Source: CAD feature listing. Evaluate the final solid. Frame: model axes, mm. Face numbers are marked on the shaded views. A direction names the side the tool comes from. Give positions to 0.01 mm unless a question says otherwise; leave off trailing zeros. Order: outer loops, then holes, each group sorted by start corner. A loop starts at its lowest first (then second) coordinate and runs counter-clockwise, first axis right, second up. Notation, with made-up numbers: M -11,50.25 L 17,50.25 A19 ccw 17,61.25 Z; hole C -31,48 d8. An arc over 180 degrees is marked long. Answer as a JSON object with one key per item and string values. Group by question number.
1. Section query B-B (x = 0). Output: boundary loops of the cut face in (y, z).
2. Pin query (flat end, axial travel): P1, Ø3, axis at x = -27, z = -22, coming from the +Y side; P2, Ø6, axis at x = 7, y = 9.5, coming from the -Z side; P3, Ø2, axis at x = 7, y = 5.5, coming from the +Z side. Return the tip coordinate at first contact, or that it passes through.
3. Section query A-A (z = 0). Output: boundary loops of the cut face in (x, y).
4. Pull-direction query (Z, two-part tool) for the marked faces 3, 4 and 5; classes: +Z half, -Z half, draft (parallel to the pull), parting line (faces both ways), or undercut.
5. Set-up query: the marked faces 1 and 2. Return all of +Z, -Z, +X, -X, +Y, -Y with unobstructed straight access to the full face (end or side cutting, diameter ignored); none if empty.
6. Section query C-C (y = 9.5). Output: boundary loops of the cut face in (x, z), plus the area to 3 significant figures.
7. Material intervals for L1, parallel to X at y = 4.25, z = -0.5; L2, parallel to Y at x = 19.5, z = 22; L3, parallel to Z at x = 7, y = 7.75, sorted ascending. Write a range as [from, to].
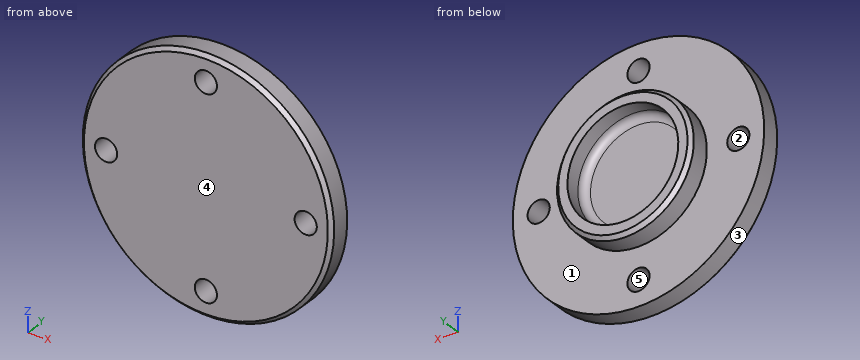
from build123d import *

# Parameters (mm, degrees)
SKETCH_1_R               = 34
EXTRUDE_1_DEPTH          = 6
SKETCH_2_R               = 18.5
SKETCH_2_R_2             = 15
EXTRUDE_2_DEPTH          = 6
SKETCH_5_R               = 3
CUT_EXTRUDE_1_DEPTH      = 6
PATTERN_CIRCULAR_1_COUNT = 4
FILLET_1_R               = 2
CHAMFER_1_SIZE           = 1


with BuildPart() as part:
    # 草图1 → 凸台-拉伸1 (new body)
    with BuildSketch(Plane(origin=(0, 0, 0), x_dir=(1, 0, 0), z_dir=(0, 1, 0))):
        with Locations(Location((0, 0, 0), (0, 0, 270))):
            Circle(SKETCH_1_R)
    extrude(amount=EXTRUDE_1_DEPTH)

    # 草图2 → 凸台-拉伸2 (add)
    with BuildSketch(Plane(origin=(0, 6, 0), x_dir=(1, 0, 0), z_dir=(0, 1, 0))):
        with Locations(Location((0, 0, 0), (0, 0, 270))):
            Circle(SKETCH_2_R)
        with Locations(Location((0, 0, 0), (0, 0, 270))):
            Circle(SKETCH_2_R_2, mode=Mode.SUBTRACT)
    extrude(amount=EXTRUDE_2_DEPTH)

    # 草图5 → 切除-拉伸1 (cut)
    with BuildSketch(Plane(origin=(0, 6, 0), x_dir=(1, 0, 0), z_dir=(0, 1, 0))):
        with Locations(Location((0, 27, 0), (0, 0, 270))):
            Circle(SKETCH_5_R)
    cut_extrude_1 = extrude(amount=-CUT_EXTRUDE_1_DEPTH, mode=Mode.SUBTRACT)

    # 阵列(圆周)1: 切除-拉伸1 ×4 about axis
    pattern_circular_1_axis = Axis((0, 0, 0), (0, 1, 0))
    for i in range(1, PATTERN_CIRCULAR_1_COUNT):
        add(cut_extrude_1.rotate(pattern_circular_1_axis, i * 360 / PATTERN_CIRCULAR_1_COUNT), mode=Mode.SUBTRACT)

    # 圆角1
    fillet_1_edges = [part.edges().sort_by_distance(p)[0] for p in [
        (0, 6, -15),
    ]]
    fillet(fillet_1_edges, radius=FILLET_1_R)

    # 倒角1
    chamfer_1_edges = [part.edges().sort_by_distance(p)[0] for p in [
        (0, 12, -18.5),
        (0, 0, -34),
    ]]
    chamfer(chamfer_1_edges, length=CHAMFER_1_SIZE)


solid = part.part
Answer sheet:
{
 "1": {"outline": "M 0,-33 L 1,-34 L 6,-34 L 6,-30 L 0,-30 Z; M 0,-24 L 6,-24 L 6,-18.5 L 11,-18.5 L 12,-17.5 L 12,-15 L 8,-15 A2 cw 6,-13 L 6,13 A2 cw 8,15 L 12,15 L 12,17.5 L 11,18.5 L 6,18.5 L 6,24 L 0,24 Z; M 0,30 L 6,30 L 6,34 L 1,34 L 0,33 Z"},
 "2": {"P1": "y = 6", "P2": "z = -18.06", "P3": "z = 33.47"},
 "3": {"outline": "M -34,1 L -33,0 L -30,0 L -30,6 L -34,6 Z; M -24,0 L 24,0 L 24,6 L 18.5,6 L 18.5,11 L 17.5,12 L 15,12 L 15,8 A2 cw 13,6 L -13,6 A2 cw -15,8 L -15,12 L -17.5,12 L -18.5,11 L -18.5,6 L -24,6 Z; M 30,0 L 33,0 L 34,1 L 34,6 L 30,6 Z"},
 "4": {"face 3": "parting line", "face 4": "draft", "face 5": "undercut"},
 "5": {"face 1": "+Y", "face 2": "+Y, -Y"},
 "6": {"outline": "C 0,0 d37; hole C 0,0 d30", "area": "368 mm^2"},
 "7": {"L1": "[-34, -29.96], [-24.04, 24.04], [29.96, 34]", "L2": "[0, 6]", "L3": "[-17.12, -13.25], [13.25, 17.12]"}
}
